Source: three-view drawing plus pictorial views. Frame: mm from the lowest corner of the part. Round coordinates to 2 decimals unless told otherwise and drop trailing zeros. Loops run counter-clockwise (first coordinate to the right, second up) from the corner with the lowest first, then second, coordinate; pieces in that order, holes last. Notation, with made-up numbers: (-0.5, 35) -> (31.5, 35) arc R10 ccw to (31.5, 53) -> close; hole circle Ø4 at (54, 64.5). An arc over 180 degrees is marked (long way). Answer as a JSON object with one key per item and string values. Group by question number.
Item 1: Section query B-B on z = 109. Return loops of the section in (x, y), and give its area (3 significant figures).
Item 2: Material intervals for line 1 (X direction, y = 1.4, z = 99); line 2 (X direction, y = 0.6, z = 5); line 3 (Z direction, x = 5, y = 1.7), sorted ascending. Write a range as [from, to].
Item 3: Section query C-C on x = 10. Return loops of the section in (y, z), and give its area (3 significant figures).
Item 4: Section query A-A on x = 147. Return loops of the section in (y, z).
Item 5: Section query D-D on y = 1.2. Return loops of the section in (x, z).
Item 6: Pin query (flat end, axial travel): pin 1 (2 mm diameter, centred on x = 147, z = 5, fed in from -Y). Return the tip coordinate at first contact, or that it passes through.
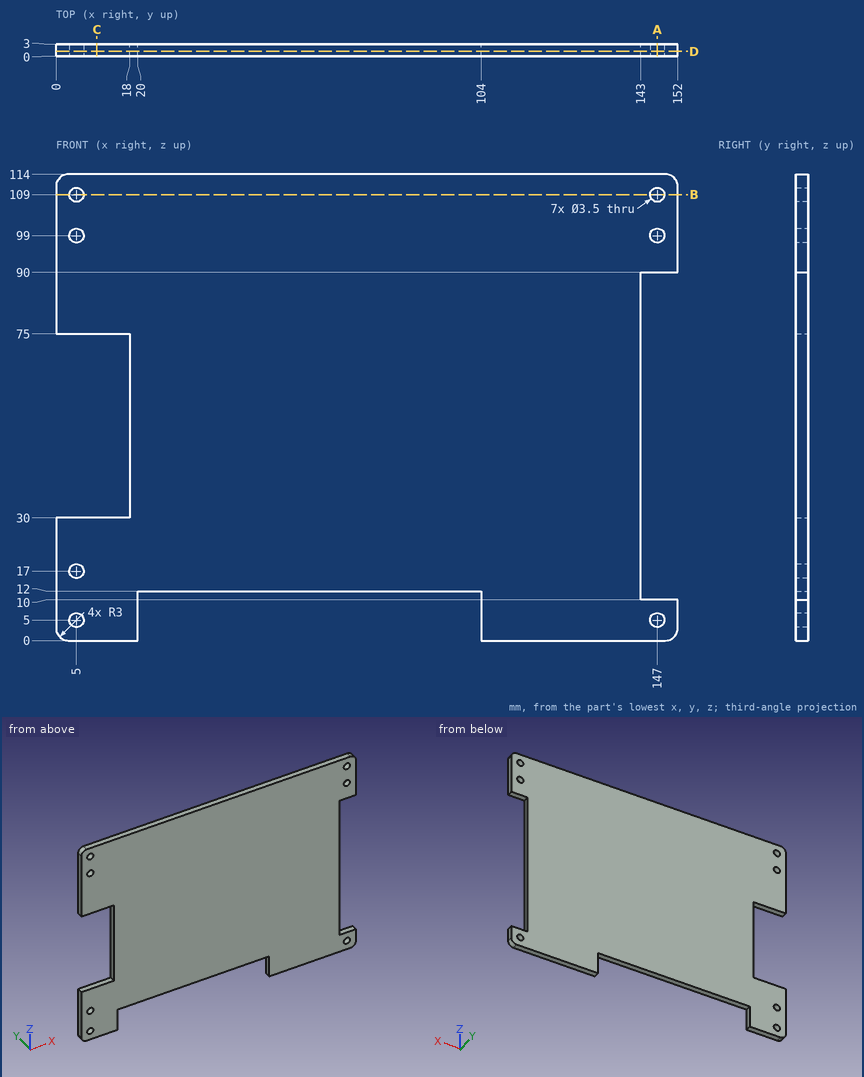
Solved:
{
 "1": {"outline": "(0, 0) -> (3.25, 0) -> (3.25, 3) -> (0, 3) -> close; (6.75, 0) -> (145.25, 0) -> (145.25, 3) -> (6.75, 3) -> close; (148.75, 0) -> (152, 0) -> (152, 3) -> (148.75, 3) -> close", "area": "435 mm²"},
 "2": {"line 1": "[0, 3.25], [6.75, 145.25], [148.75, 152]", "line 2": "[0, 3.25], [6.75, 20], [104, 145.25], [148.75, 152]", "line 3": "[0, 3.25], [6.75, 15.25], [18.75, 30], [75, 97.25], [100.75, 107.25], [110.75, 114]"},
 "3": {"outline": "(0, 0) -> (3, 0) -> (3, 30) -> (0, 30) -> close; (0, 75) -> (3, 75) -> (3, 114) -> (0, 114) -> close", "area": "207 mm²"},
 "4": {"outline": "(0, 0) -> (3, 0) -> (3, 3.25) -> (0, 3.25) -> close; (0, 6.75) -> (3, 6.75) -> (3, 10) -> (0, 10) -> close; (0, 90) -> (3, 90) -> (3, 97.25) -> (0, 97.25) -> close; (0, 100.75) -> (3, 100.75) -> (3, 107.25) -> (0, 107.25) -> close; (0, 110.75) -> (3, 110.75) -> (3, 114) -> (0, 114) -> close"},
 "5": {"outline": "(0, 3) arc R3 ccw to (3, 0) -> (20, 0) -> (20, 12) -> (104, 12) -> (104, 0) -> (149, 0) arc R3 ccw to (152, 3) -> (152, 10) -> (143, 10) -> (143, 90) -> (152, 90) -> (152, 111) arc R3 ccw to (149, 114) -> (3, 114) arc R3 ccw to (0, 111) -> (0, 75) -> (18, 75) -> (18, 30) -> (0, 30) -> close; hole circle Ø3.5 at (5, 5); hole circle Ø3.5 at (5, 17); hole circle Ø3.5 at (5, 99); hole circle Ø3.5 at (5, 109); hole circle Ø3.5 at (147, 5); hole circle Ø3.5 at (147, 99); hole circle Ø3.5 at (147, 109)"},
 "6": {"pin 1": "through"}
}
